Geometry: see drawing. Coordinates: mm, zero at the bounding-box minimum. Coordinates: 2 decimals unless noted, no trailing zeros. Order: outer loops, then holes, each group sorted by start corner. A loop starts at its lowest first (then second) coordinate and runs counter-clockwise, first axis right, second up.
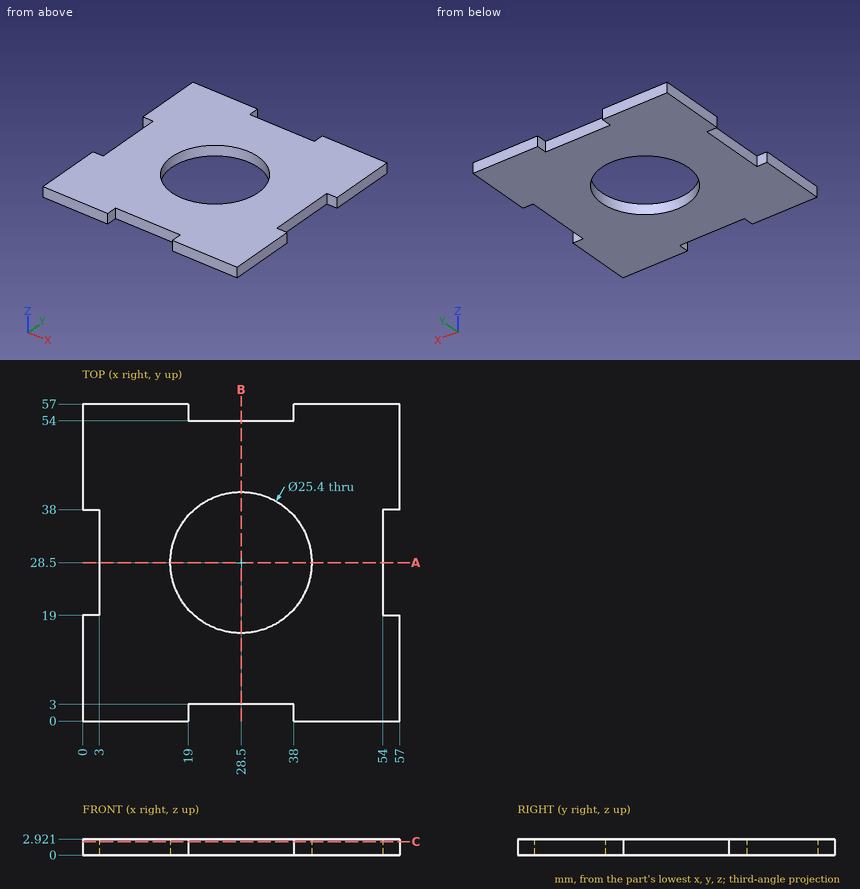
Q1. Pin query (flat end, axial travel): P1, Ø0.9, axis at y = 32, z = 1, coming from the -X side; P2, Ø0.9, axis at x = 31, z = 1.5, coming from the +Y side; P3, Ø0.9, axis at y = 32.5, z = 1, coming from the +X side. Return the tip coordinate at first contact, or that it passes through.
Solutions:
P1: stops at x = 3
P2: stops at y = 54
P3: stops at x = 54
Q2. Section query C-C on z = 2.45. Output: boundary loops of the cut face in (x, y), plus the area to 3 significant figures.
Solutions:
outline: (0, 0) - (19, 0) - (19, 3) - (38, 3) - (38, 0) - (57, 0) - (57, 19) - (54, 19) - (54, 38) - (57, 38) - (57, 57) - (38, 57) - (38, 54) - (19, 54) - (19, 57) - (0, 57) - (0, 38) - (3, 38) - (3, 19) - (0, 19) - close; hole circle Ø25.4 at (28.5, 28.5)
area: 2,510 mm2
Q3. Section query A-A on y = 28.5. Output: boundary loops of the cut face in (x, z), plus the area to 3 significant figures.
Solutions:
outline: (3, 0) - (15.8, 0) - (15.8, 2.92) - (3, 2.92) - close; (41.2, 0) - (54, 0) - (54, 2.92) - (41.2, 2.92) - close
area: 74.8 mm2
Q4. Material intervals for line 1 along X through (y, z) = (28.5, 1.05); line 2 along X through (y, z) = (32.5, 0.95); line 3 along Y through (x, z) = (21, 0.1), sorted ascending.
Solutions:
line 1: x = 3 to 15.8, 41.2 to 54
line 2: x = 3 to 16.45, 40.55 to 54
line 3: y = 3 to 18.25, 38.75 to 54
